Could you check a few things on this drawing? It's one solid part, dimensions in mm from its lowest x, y, z. A direction names the side the tool comes from. Coordinates: 2 decimals unless noted, no trailing zeros. Loops run counter-clockwise (first coordinate to the right, second up) from the corner with the lowest first, then second, coordinate; pieces in that order, holes last. Notation, with made-up numbers: M -40,79 L -13,79 A11 ccw -13,87 Z; hole C 1.25,70 d7. An arc over 180 degrees is marked long. Answer as a JSON object with one key per item and string values. Group by question number.
Item 1: If I drill on line 1 (Z direction, x = 68, y = 455); line 2 (Z direction, x = 35, y = 2); line 3 (X direction, y = 2, z = 32) (1 decimal), over which ranges is the centre line in solid material (lowest first)?
Item 2: Suppose I cut it at D-D (x = 14). Write out the boundary of the cut face in (y, z).
Item 3: Suppose I cut it at C-C (z = 61). Write out the boundary of the cut face in (x, y), then the cut area to 3 significant figures.
Item 4: I'm going to push flat-ended pins straight in: pin 1 Ø10 at (x, z) = (59.5, 108) entering from +Y; pin 2 Ø12 at (y, z) = (299, 42.5) entering from -X. Where does each tip first touch, or does it pass through?
Item 5: Which directions (+Z, -Z, +X, -X, +Y, -Y) give clear straight access to the entire face, cutting with the end or side of a thin tool? Please do the marked faces 1 and 2.
Item 6: Suppose I cut it at A-A (y = 455). Write out the boundary of the cut face in (x, z).
Item 7: Suppose I cut it at B-B (z = 32.5). Write out the boundary of the cut face in (x, y).
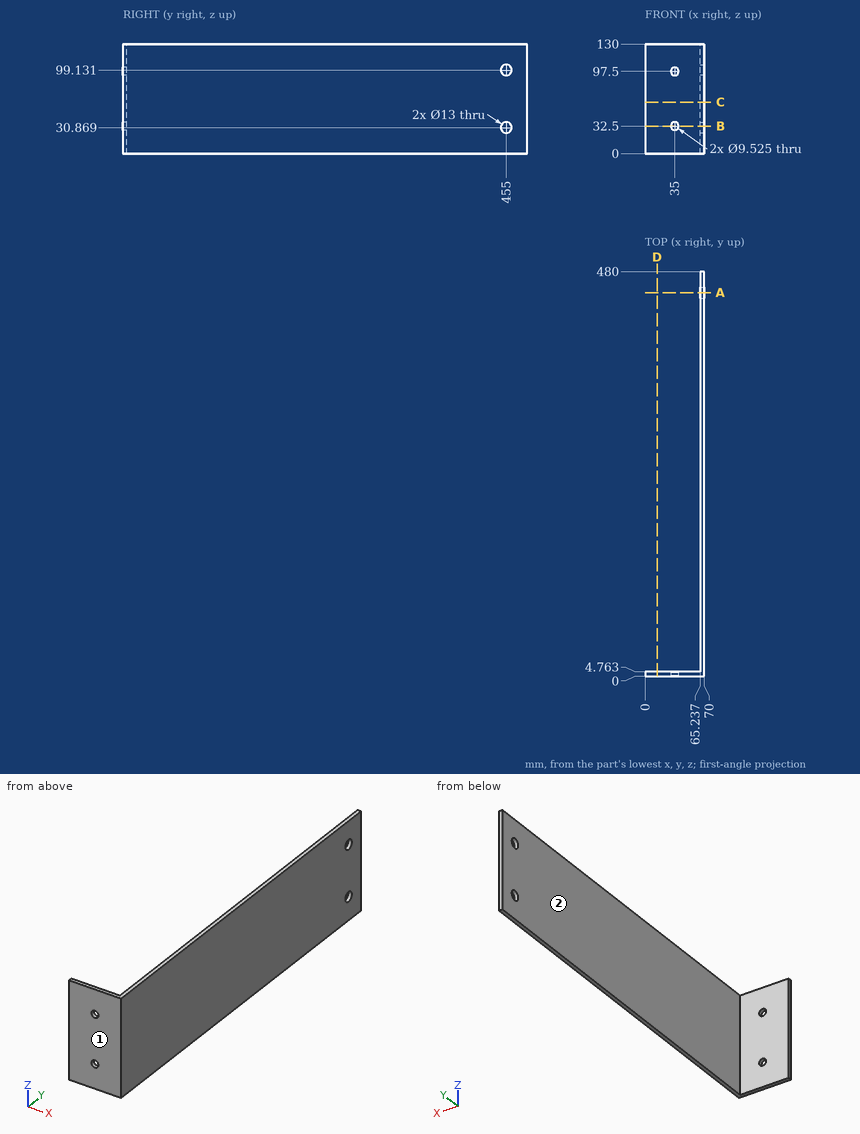
From the geometry:
{
 "1": {"line 1": "0 to 24.37, 37.37 to 92.63, 105.63 to 130", "line 2": "0 to 27.74, 37.26 to 92.74, 102.26 to 130", "line 3": "0 to 30.3, 39.7 to 70"},
 "2": {"outline": "M 0,0 L 4.76,0 L 4.76,130 L 0,130 Z"},
 "3": {"outline": "M 0,0 L 70,0 L 70,480 L 65.24,480 L 65.24,4.76 L 0,4.76 Z", "area": "2,600 mm2"},
 "4": {"pin 1": "y = 4.76", "pin 2": "x = 65.24"},
 "5": {"face 1": "+Z, -Z, +X, -X, -Y", "face 2": "+Z, -Z, -X, +Y"},
 "6": {"outline": "M 65.24,0 L 70,0 L 70,24.37 L 65.24,24.37 Z; M 65.24,37.37 L 70,37.37 L 70,92.63 L 65.24,92.63 Z; M 65.24,105.63 L 70,105.63 L 70,130 L 65.24,130 Z"},
 "7": {"outline": "M 0,0 L 30.24,0 L 30.24,4.76 L 0,4.76 Z; M 39.76,0 L 70,0 L 70,448.71 L 65.24,448.71 L 65.24,4.76 L 39.76,4.76 Z; M 65.24,461.29 L 70,461.29 L 70,480 L 65.24,480 Z"}
}
